Check sheet for the modelled part. Datum: model origin and axes. Units: mm. A direction names the side the tool comes from. Round coordinates to 2 decimals unless told otherwise and drop trailing zeros. Write each loop counter-clockwise with the first axis right and the second up, starting at its lowest first coordinate (ties: lowest second). Pieces come first, ordered by that corner, then holes. Notation, with made-up numbers: (79, 59) - (86, 59) arc R8 cw to (86, 63) - close; hole circle Ø1 at (-15, -7.75). An arc over 180 degrees is marked (long way). Answer as a JSON object with one key per item and string values. Group by question number.
Item 1: Set-up check for faces 1 (the cylindrical face through (1.47, -0.78, 2.83)), 2 (the flat face through (4.207, 1.565, 7.425)): record each of +Z, -Z, +X, -X, +Y, -Y from which the full face is reachable in a straight line by a thin tool's end or side.
Item 2: Release check for a two-part mould opening along X. For faces 3 (the flat face through (4, 3.175, -8)), 4 (the flat face through (4.327, 1.565, -7.357)), 5 (the cylindrical face through (10.914, 0.827, -3.437)), 6 (the flat face through (-8.534, 2, 0)) record: pulls with the +X half, pulls with the -X half, needs draft (parallel to the pull), parting line crosses it, or undercut.
Item 3: Sectioned sample at B-B on y = 1.55. Record the boundary of the cut face in (x, z).
Item 4: Sectioned sample at D-D on z = 4. Record the boundary of the cut face in (x, y) (1 decimal).
Item 5: Sectioned sample at A-A on z = 0. Record the boundary of the cut face in (x, y) (1 decimal).
Item 6: Gauge pin test, flat ends, axial feed: P1, Ø5, axis at x = 1, z = 0, coming from the +Y side; P2, Ø2, axis at y = -1, z = -4.5, coming from the -X side; P3, Ø1, axis at y = 1, z = -1.5, coming from the -X side; P4, Ø5, axis at x = 0, z = 0, coming from the +Y side. Record the tip position at first contact, or that the pin passes through.
Item 7: Sectioned sample at C-C on x = 2.75. Record the boundary of the cut face in (y, z) (1 decimal), plus the area to 3 significant figures.
Item 8: Thickness scan on line 1 (Z direction, x = 0, y = -1.2); line 2 (Y direction, x = -3, z = 6.25). Record the ranges inside material, lowest first.
```python
from build123d import *

# Parameters (mm, degrees)
SKETCH1_R           = 11.442176275
BOSS_EXTRUDE1_DEPTH = 3.175
SKETCH2_R           = 11.442176275
SKETCH2_R_2         = 3.1877
BOSS_EXTRUDE2_DEPTH = 1.5875


with BuildPart() as part:
    # Sketch1 → Boss-Extrude1 (new body)
    with BuildSketch(Plane(origin=(0, 0, 0), x_dir=(1, 0, 0), z_dir=(0, 1, 0))):
        Circle(SKETCH1_R)
        Polygon((8.5344, 4.927338137), (0, 9.854676275), (-8.5344, 4.927338137), (-8.5344, -4.927338137), (0, -9.854676275), (8.5344, -4.927338137), align=None, mode=Mode.SUBTRACT)
    extrude(amount=BOSS_EXTRUDE1_DEPTH)

    # Sketch2 → Boss-Extrude2 (add)
    with BuildSketch(Plane(origin=(0, 0, 0), x_dir=(1, 0, 0), z_dir=(0, 1, 0))):
        Circle(SKETCH2_R)
        Circle(SKETCH2_R_2, mode=Mode.SUBTRACT)
    extrude(amount=-BOSS_EXTRUDE2_DEPTH)


solid = part.part
```
Completed:
{
 "1": {"face 1": "+Y, -Y", "face 2": "+Y"},
 "2": {"face 3": "needs draft", "face 4": "undercut", "face 5": "parting line crosses it", "face 6": "undercut"},
 "3": {"outline": "circle Ø22.88 at (0, 0); hole (-8.53, -4.93) - (0, -9.85) - (8.53, -4.93) - (8.53, 4.93) - (0, 9.85) - (-8.53, 4.93) - close"},
 "4": {"outline": "(-10.7, -1.6) - (10.7, -1.6) - (10.7, 3.2) - (8.5, 3.2) - (8.5, 0) - (-8.5, 0) - (-8.5, 3.2) - (-10.7, 3.2) - close"},
 "5": {"outline": "(-11.4, -1.6) - (-3.2, -1.6) - (-3.2, 0) - (-8.5, 0) - (-8.5, 3.2) - (-11.4, 3.2) - close; (3.2, -1.6) - (11.4, -1.6) - (11.4, 3.2) - (8.5, 3.2) - (8.5, 0) - (3.2, 0) - close"},
 "6": {"P1": "y = 0", "P2": "x = -10.89", "P3": "x = -11.4", "P4": "through"},
 "7": {"outline": "(-1.6, -11.1) - (3.2, -11.1) - (3.2, -8.3) - (0, -8.3) - (0, -1.6) - (-1.6, -1.6) - close; (-1.6, 1.6) - (0, 1.6) - (0, 8.3) - (3.2, 8.3) - (3.2, 11.1) - (-1.6, 11.1) - close", "area": "48.2 mm²"},
 "8": {"line 1": "-11.44 to -3.19, 3.19 to 11.44", "line 2": "-1.59 to 0"}
}
